```python
from build123d import *

# Parameters (mm, degrees)
PAD_DEPTH            = 10
SKETCH001_R          = 28.1
SKETCH001_R_2        = 1.5
POCKET_DEPTH         = 4.5
POCKET001_DEPTH      = 62.501
POCKET001_DEPTH_BACK = -62.501
HOLE_D               = 5
HOLE_DEPTH           = 25
HOLE_CSINK_D         = 10
HOLE_CSINK_ANGLE     = 90
SKETCH005_W          = 5
SKETCH005_H          = 6
PAD001_DEPTH         = 4
POCKET002_DEPTH      = 42.5
CHAMFER_SIZE         = 3.5
FILLET_R             = 3.5


with BuildPart() as part:
    # Sketch → Pad (new body)
    with BuildSketch(Plane.XY):
        with BuildLine():
            Line((-48.25, -48.4), (-40.5, -48.4))
            ThreePointArc((-38.25, -50.65), (-38.90901, -49.05901), (-40.5, -48.4))
            Line((-38.25, -50.65), (-38.25, -51.4))
            Line((-38.25, -51.4), (38.25, -51.4))
            Line((38.25, -51.4), (38.25, -50.65))
            ThreePointArc((40.5, -48.4), (38.90901, -49.05901), (38.25, -50.65))
            Line((40.5, -48.4), (48.25, -48.4))
            Line((48.25, -48.4), (62.5, -62.65))
            Line((62.5, -62.65), (62.5, -146.4))
            Line((57.5, -151.4), (62.5, -146.4))
            Line((-57.5, -151.4), (57.5, -151.4))
            Line((-62.5, -146.4), (-57.5, -151.4))
            Line((-62.5, -146.4), (-62.5, -62.65))
            Line((-62.5, -62.65), (-48.25, -48.4))
        make_face()
    extrude(amount=PAD_DEPTH)

    # Sketch001 → Pocket (cut)
    with BuildSketch(Plane.XY.offset(10)):
        with Locations((-30, -116.4)):
            Circle(SKETCH001_R)
        with Locations((30, -116.4)):
            Circle(SKETCH001_R)
        with Locations((-37.5, -85.4)):
            Circle(SKETCH001_R_2)
        with Locations((-22.5, -85.4)):
            Circle(SKETCH001_R_2)
        with Locations((22.5, -85.4)):
            Circle(SKETCH001_R_2)
        with Locations((37.5, -85.4)):
            Circle(SKETCH001_R_2)
        with Locations((-37.5, -147.4)):
            Circle(SKETCH001_R_2)
        with Locations((-22.5, -147.4)):
            Circle(SKETCH001_R_2)
        with Locations((22.5, -147.4)):
            Circle(SKETCH001_R_2)
        with Locations((37.5, -147.4)):
            Circle(SKETCH001_R_2)
    extrude(amount=-POCKET_DEPTH, mode=Mode.SUBTRACT)

    # Sketch002 → Pocket001 (cut, two sides)
    with BuildSketch(Plane.YZ) as pocket001_sk:
        Polygon((0, 2), (-65, 2), (-85, 22), (0, 22), align=None)
    extrude(amount=-POCKET001_DEPTH, mode=Mode.SUBTRACT)
    extrude(pocket001_sk.sketch, amount=-POCKET001_DEPTH_BACK, mode=Mode.SUBTRACT)

    # Hole
    with Locations(Plane.XY.offset(10)):
        with Locations((-55, -91.4), (55, -91.4), (55, -141.4), (-55, -141.4)):
            CounterSinkHole(HOLE_D / 2, HOLE_CSINK_D / 2, depth=HOLE_DEPTH, counter_sink_angle=HOLE_CSINK_ANGLE)

    # Sketch005 (on Face6 of Hole) → Pad001 (join)
    with BuildSketch(Plane.XY.offset(10)):
        with Locations((-36.5, -77.4)):
            Rectangle(SKETCH005_W, SKETCH005_H)
        with Locations((-23.5, -77.4)):
            Rectangle(SKETCH005_W, SKETCH005_H)
        with Locations((23.5, -77.4)):
            Rectangle(SKETCH005_W, SKETCH005_H)
        with Locations((36.5, -77.4)):
            Rectangle(SKETCH005_W, SKETCH005_H)
    extrude(amount=PAD001_DEPTH)

    # Sketch006 → Pocket002 (cut, symmetric)
    with BuildSketch(Plane.YZ):
        with BuildLine():
            ThreePointArc((-54.131371, 0.868629), (-53, 0.4), (-51.868629, 0.868629))
            Line((-51.868629, 0.868629), (-37.737258, 15))
            Line((-68.262742, 15), (-37.737258, 15))
            Line((-54.131371, 0.868629), (-68.262742, 15))
        make_face()
    extrude(amount=POCKET002_DEPTH, both=True, mode=Mode.SUBTRACT)

    # Chamfer
    chamfer_edges = [part.edges().sort_by_distance(p)[0] for p in [
        (39, -77.4, 14),
        (21, -77.4, 14),
        (-21, -77.4, 14),
        (-39, -77.4, 14),
    ]]
    chamfer(chamfer_edges, length=CHAMFER_SIZE)

    # Fillet
    fillet_edges = [part.edges().sort_by_distance(p)[0] for p in [
        (-34, -77.4, 10),
        (26, -77.4, 10),
        (-26, -77.4, 10),
        (34, -77.4, 10),
    ]]
    fillet(fillet_edges, radius=FILLET_R)


solid = part.part
```
Input: part model. Units: mm. Frame: model coordinates. A direction names the side the tool comes from. Coordinates: 2 decimals unless noted, no trailing zeros. Write each loop counter-clockwise with the first axis right and the second up, starting at its lowest first coordinate (ties: lowest second). Pieces come first, ordered by that corner, then holes. Notation, with made-up numbers: (54, -39.5) -> (93, -39.5) arc R24 ccw to (93, -8.5) -> close; hole circle Ø6 at (82, -4). An arc over 180 degrees is marked (long way). Write each question's results on one line, items separated by ' | '.
Item 1: Section query D-D on x = 22.5. Return loops of the section in (y, z).
Conclusion:
outline: (-151.4, 0) -> (-51.4, 0) -> (-51.4, 1.34) -> (-51.87, 0.87) arc R1.6 cw to (-54.13, 0.87) -> (-55.26, 2) -> (-65, 2) -> (-73, 10) -> (-74.4, 10) -> (-74.4, 12) -> (-80.4, 12) -> (-80.4, 10) -> (-83.9, 10) -> (-83.9, 5.5) -> (-86.9, 5.5) -> (-86.9, 10) -> (-89.32, 10) -> (-89.32, 5.5) -> (-143.48, 5.5) -> (-143.48, 10) -> (-145.9, 10) -> (-145.9, 5.5) -> (-148.9, 5.5) -> (-148.9, 10) -> (-151.4, 10) -> close
Item 2: Set-up query: faces 1 (the cylindrical face through (-27.05, -77.36, 11)), 2 (the flat face through (36, -74.4, 12)), 3 (the flat face through (-38, -85, 5.5)). Return all of +Z, -Z, +X, -X, +Y, -Y with unobstructed straight access to the full face (end or side cutting, diameter ignored); none if empty.
Conclusion:
face 1: +Z, +Y, -Y | face 2: +Z, +X, -X, +Y | face 3: +Z
Item 3: Section query C-C on y = -141.4. Return loops of the section in (x, z), plus the area to 3 significant figures.
Conclusion:
outline: (-62.5, 0) -> (-57.5, 0) -> (-57.5, 7.5) -> (-60, 10) -> (-62.5, 10) -> close; (-52.5, 0) -> (52.5, 0) -> (52.5, 7.5) -> (50, 10) -> (42.83, 10) -> (42.83, 5.5) -> (17.17, 5.5) -> (17.17, 10) -> (-17.17, 10) -> (-17.17, 5.5) -> (-42.83, 5.5) -> (-42.83, 10) -> (-50, 10) -> (-52.5, 7.5) -> close; (57.5, 0) -> (62.5, 0) -> (62.5, 10) -> (60, 10) -> (57.5, 7.5) -> close | area: 907 mm^2
Item 4: Mould query, pull axis X, two halves, no side actions, for faces 4 (the flat face through (-24, -80.4, 12)), 5 (the flat face through (62.5, -104, 5)), 6 (the cylindrical face through (22.175, -86.864, 7.781)). Classes: +X half, -X half, draft (parallel to the pull), parting line (faces both ways), or undercut.
Conclusion:
face 4: draft | face 5: +X half | face 6: undercut
Item 5: Pin query (flat end, axial travel): pin 1 Ø5 at (x, y) = (-24.5, -68) entering from +Z; pin 2 Ø1.2 at (x, z) = (35, 11.5) entering from -Y; pin 3 Ø1 at (x, y) = (47.5, -132.5) entering from +Z. Return the tip coordinate at first contact, or that it passes through.
Conclusion:
pin 1: stops at z = 7.5 | pin 2: stops at y = -80.4 | pin 3: stops at z = 5.5
Item 6: Material intervals for probe 1 along X at (y, z) = (-118, 8.25); probe 2 along X at (y, z) = (-96, 6); probe 3 along X at (y, z) = (-147.4, 7.1), sorted ascending.
Conclusion:
probe 1: x = -62.5 to -58.05, -1.95 to 1.95, 58.05 to 62.5 | probe 2: x = -62.5 to -49.32, -10.68 to 10.68, 49.32 to 62.5 | probe 3: x = -61.5 to -39, -36 to -24, -21 to 21, 24 to 36, 39 to 61.5
Item 7: Section query B-B on z = 12. Return loops of the section in (x, y), plus the area to 3 significant figures.
Conclusion:
outline: (-37.5, -80.4) -> (-33.66, -80.4) -> (-33.66, -74.4) -> (-37.5, -74.4) -> close; (-26.34, -80.4) -> (-22.5, -80.4) -> (-22.5, -74.4) -> (-26.34, -74.4) -> close; (22.5, -80.4) -> (26.34, -80.4) -> (26.34, -74.4) -> (22.5, -74.4) -> close; (33.66, -80.4) -> (37.5, -80.4) -> (37.5, -74.4) -> (33.66, -74.4) -> close | area: 92.1 mm^2
Item 8: Section query A-A on x = -55. Return loops of the section in (y, z).
Conclusion:
outline: (-151.4, 0) -> (-143.9, 0) -> (-143.9, 7.5) -> (-146.4, 10) -> (-151.4, 10) -> close; (-138.9, 0) -> (-93.9, 0) -> (-93.9, 7.5) -> (-96.4, 10) -> (-103.57, 10) -> (-103.57, 5.5) -> (-129.23, 5.5) -> (-129.23, 10) -> (-136.4, 10) -> (-138.9, 7.5) -> close; (-88.9, 0) -> (-55.15, 0) -> (-55.15, 2) -> (-65, 2) -> (-73, 10) -> (-86.4, 10) -> (-88.9, 7.5) -> close
